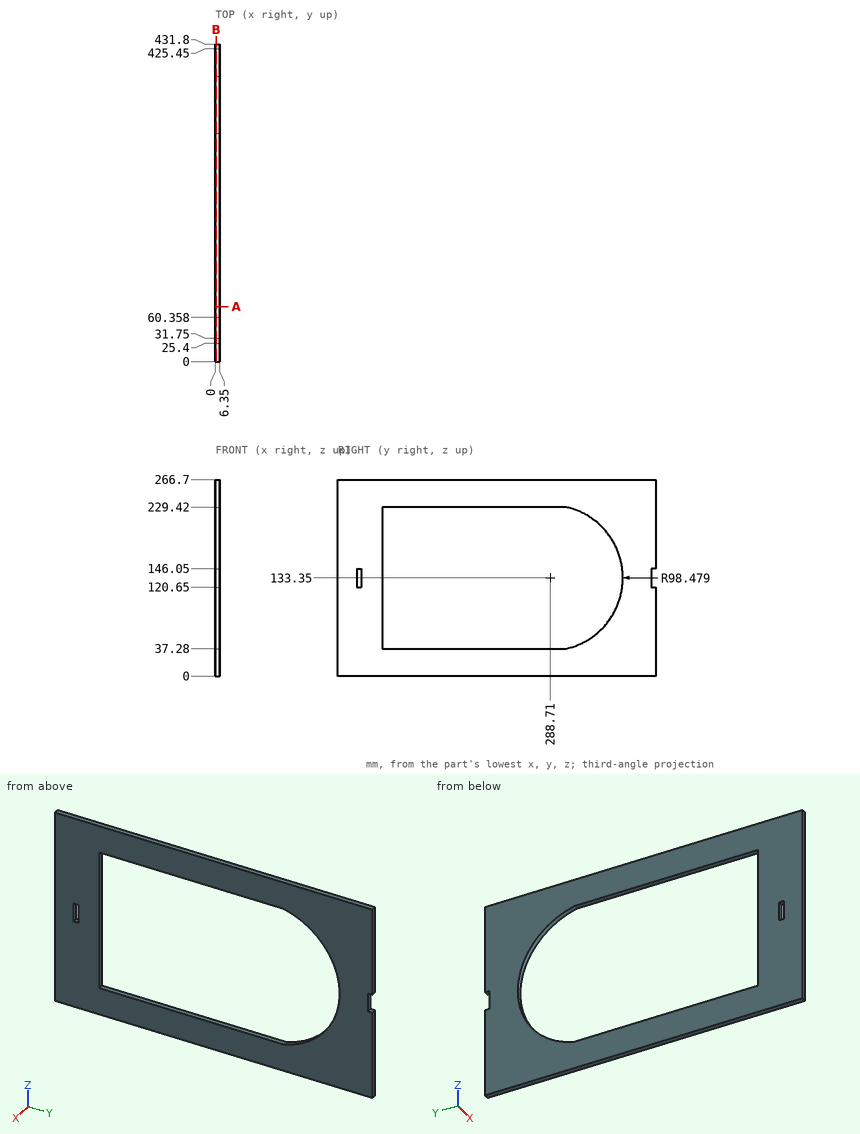
Job drawing, mm, ordinate dimensions from the low corner. One solid piece. Round coordinates to 2 decimals unless told otherwise and drop trailing zeros. Write each loop counter-clockwise with the first axis right and the second up, starting at its lowest first coordinate (ties: lowest second). Pieces come first, ordered by that corner, then holes.
1) Band-saw the part on B-B, the plane x = 1. List the corners of the cut face in (y, z), and give its area (3 significant figures).
2) Band-saw the part on A-A, the plane y = 75. List the corners of the cut face in (x, z).
3) Pin check, flat tip, straight feed: pin 1 (3 mm diameter, centred on x = 4, z = 130.5, fed in from +Y). Stop position of the tip, or through.
4) Drill centre lines: probe 1 along Z at (x, y) = (2, 92.5); probe 2 along Y at (x, z) = (1.5, 131); probe 3 along Y at (x, z) = (2, 157.5). Where is each one in solid material? Low to high.
Ans:
1. outline: (0, 0) - (431.8, 0) - (431.8, 120.65) - (425.45, 120.65) - (425.45, 146.05) - (431.8, 146.05) - (431.8, 266.7) - (0, 266.7) - close; hole (25.4, 120.65) - (31.75, 120.65) - (31.75, 146.05) - (25.4, 146.05) - close; hole (60.36, 37.28) - (310.36, 37.28) arc R98.48 ccw to (310.36, 229.42) - (60.36, 229.42) - close
1. area: 55,800 mm2
2. outline: (0, 0) - (6.35, 0) - (6.35, 37.28) - (0, 37.28) - close; (0, 229.42) - (6.35, 229.42) - (6.35, 266.7) - (0, 266.7) - close
3. pin 1: stops at y = 425.45
4. probe 1: z = 0 to 37.28, 229.42 to 266.7
4. probe 2: y = 0 to 25.4, 31.75 to 60.36, 387.16 to 425.45
4. probe 3: y = 0 to 60.36, 384.18 to 431.8
